```python
from build123d import *

# Parameters (mm, degrees)
F1_DEPTH  = 55
F2_W      = 5
F2_H      = 4
F3_DEPTH  = 110.001
F4_R      = 6
F5_DEPTH  = 20
F6_R      = 6
F7_DEPTH  = 20
F9_DEPTH  = 110.001
F10_SIZE2 = 4.041452
F10_SIZE  = 7
F11_R     = 2
F12_DEPTH = 55.001


with BuildPart() as f1:
    # F0 (on Front) → F1 (new body)
    with BuildSketch(Plane.XZ):
        Polygon((-45.460895, 50), (-45.460895, 0), (-35.460895, 0), (-35.460895, 34), (54.539105, 34), (54.539105, 0), (64.539105, 0), (64.539105, 50), align=None)
    extrude(amount=F1_DEPTH)

    # F2 (on face) → F3 (cut, through all)
    with BuildSketch(Plane(origin=(-45.460895, 0, 0), x_dir=(0, -1, 0), z_dir=(-1, 0, 0))):
        with Locations((2.5, 2)):
            Rectangle(F2_W, F2_H)
        with Locations((52.5, 2)):
            Rectangle(F2_W, F2_H)
    extrude(amount=-F3_DEPTH, mode=Mode.SUBTRACT)

    # F4 (on face) → F5 (join)
    with BuildSketch(Plane(origin=(-45.460895, 0, 0), x_dir=(0, -1, 0), z_dir=(-1, 0, 0))):
        with Locations((27.5, 11)):
            Circle(F4_R)
    extrude(amount=F5_DEPTH)

    # F6 (on face) → F7 (join)
    with BuildSketch(Plane(origin=(54.539105, 0, 0), x_dir=(0, -1, 0), z_dir=(-1, 0, 0))):
        with Locations((27.5, 11)):
            Circle(F6_R)
    extrude(amount=F7_DEPTH)

    # F8 (on face) → F9 (cut, through all)
    with BuildSketch(Plane(origin=(-45.460895, 0, 0), x_dir=(0, -1, 0), z_dir=(-1, 0, 0))):
        Polygon((40, 32.825176), (55, 27), (55, 50), (40, 50), align=None)
        Polygon((15, 32.825176), (15, 50), (0, 50), (0, 27), align=None)
    extrude(amount=-F9_DEPTH, mode=Mode.SUBTRACT)

    # F10
    f10_edges = [f1.edges().sort_by_distance(p)[0] for p in [
        (-65.460895, -21.5, 11),
        (34.539105, -21.5, 11),
    ]]
    chamfer(f10_edges, length=F10_SIZE, length2=F10_SIZE2)

    # F11 (on Front) → F12 (cut, through all)
    with BuildSketch(Plane.XZ):
        with Locations((-53.460895, 17)):
            Circle(F11_R)
        with Locations((46.539105, 17)):
            Circle(F11_R)
    extrude(amount=F12_DEPTH, mode=Mode.SUBTRACT)


solid = f1.part
```
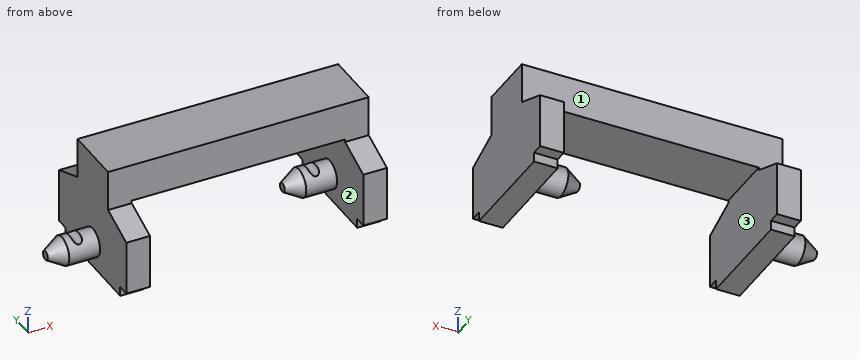
Geometry: final body of the model. Coordinates: model frame, mm. Face numbers are marked on the shaded views. A direction names the side the tool comes from. Round coordinates to 2 decimals unless told otherwise and drop trailing zeros. Write each loop counter-clockwise with the first axis right and the second up, starting at its lowest first coordinate (ties: lowest second). Pieces come first, ordered by that corner, then holes.
Item 1: Section query A-A (x = -39). Return loops of the section in (y, z), plus the area to 3 significant figures.
Item 2: Section query C-C (y = -27.5). Return loops of the section in (x, z), plus the area to 3 significant figures.
Item 3: Section query B-B (z = 11). Return loops of the section in (x, y), plus the area to 3 significant figures.
Item 4: Material intervals for L1, parallel to X at y = -40.5, z = 8.5; L2, parallel to Z at x = 0, y = -34.5; L3, parallel to Y at x = -3.5, z = 48.5, sorted ascending.
Item 5: Pin query (flat end, axial travel): P1, Ø5.5, axis at x = -39, y = -1.5, coming from the -Z side; P2, Ø2, axis at x = -41, z = 2.5, coming from the +Y side; P3, Ø1.5, axis at x = -15.5, y = -39, coming from the -Z side; P4, Ø5, axis at x = 28, y = -10.5, coming from the +Z side. Return the tip coordinate at first contact, or that it passes through.
Item 6: Section query D-D (y = -43). Return loops of the section in (x, z), plus the area to 3 significant figures.
Item 7: Set-up query: the marked faces 1, 2 and 3. Return all of +Z, -Z, +X, -X, +Y, -Y with unobstructed straight access to the full face (end or side cutting, diameter ignored); none if empty.
Completed:
1. outline: (-55, 4) - (-50, 4) - (-50, 0) - (-5, 0) - (-5, 4) - (0, 4) - (0, 27) - (-15, 32.83) - (-15, 50) - (-40, 50) - (-40, 32.83) - (-55, 27) - close
1. area: 2,110 mm2
2. outline: (-65.46, 9.04) - (-58.46, 5) - (-45.46, 5) - (-45.46, 0) - (-35.46, 0) - (-35.46, 34) - (54.54, 34) - (54.54, 17) - (48.54, 17) arc R2 cw to (44.54, 17) - (41.54, 17) - (34.54, 12.96) - (34.54, 9.04) - (41.54, 5) - (54.54, 5) - (54.54, 0) - (64.54, 0) - (64.54, 50) - (-45.46, 50) - (-45.46, 17) - (-51.46, 17) arc R2 cw to (-55.46, 17) - (-58.46, 17) - (-65.46, 12.96) - close
2. area: 2,850 mm2
3. outline: (-65.46, -29.46) - (-58.46, -33.5) - (-45.46, -33.5) - (-45.46, -55) - (-35.46, -55) - (-35.46, 0) - (-45.46, 0) - (-45.46, -21.5) - (-58.46, -21.5) - (-65.46, -25.54) - close; (34.54, -29.46) - (41.54, -33.5) - (54.54, -33.5) - (54.54, -55) - (64.54, -55) - (64.54, 0) - (54.54, 0) - (54.54, -21.5) - (41.54, -21.5) - (34.54, -25.54) - close
3. area: 1,520 mm2
4. L1: x = -45.46 to -35.46, 54.54 to 64.54
4. L2: z = 34 to 50
4. L3: y = -40 to -15
5. P1: stops at z = 4
5. P2: stops at y = -5
5. P3: stops at z = 34
5. P4: passes through
6. outline: (-45.46, 0) - (-35.46, 0) - (-35.46, 31.66) - (-45.46, 31.66) - close; (54.54, 0) - (64.54, 0) - (64.54, 31.66) - (54.54, 31.66) - close
6. area: 633 mm2
7. face 1: +Z, +X, -X, +Y
7. face 2: none
7. face 3: -Z, +Y, -Y
